from build123d import *

# Parameters (mm, degrees)
F0_W      = 56
F0_H      = 87.6
F1_DEPTH  = 5
F2_SIZE   = 2
F3_W      = 15.5
F3_H      = 25
F4_DEPTH  = 2.7
F5_R      = 3
F7_W      = 50
F7_H      = 81.6
F8_DEPTH  = 1.5
F9_R      = 1
F10_D     = 2.5
F10_DEPTH = 68
F10_START = 1.5
F10_TIP   = 0.7510757738


with BuildPart() as f1:
    # F0 (on Top) → F1 (new body)
    with BuildSketch(Plane.XY):
        Rectangle(F0_W, F0_H)
    extrude(amount=F1_DEPTH)

    # F2
    f2_edges = [f1.edges().sort_by_distance(p)[0] for p in [
        (-28, 0, 0),
    ]]
    chamfer(f2_edges, length=F2_SIZE)

    # F3 (on face) → F4 (cut)
    with BuildSketch(Plane.XY.offset(5)):
        Polygon((12.5, 43.8), (-12.5, 43.8), (-12.5, -43.8), (12.5, -43.8), (12.5, -12.5), (12.5, 12.5), align=None)
        with Locations((20.25, 0)):
            Rectangle(F3_W, F3_H)
    extrude(amount=-F4_DEPTH, mode=Mode.SUBTRACT)

    # F5
    f5_edges = [f1.edges().sort_by_distance(p)[0] for p in [
        (-28, 43.8, 3.5),
        (-28, -43.8, 3.5),
        (28, -43.8, 2.5),
        (28, 43.8, 2.5),
    ]]
    fillet(f5_edges, radius=F5_R)

    # F7 (on offset) → F8 (cut)
    with BuildSketch(Plane.XY.offset(5)):
        Rectangle(F7_W, F7_H)
    extrude(amount=-F8_DEPTH, mode=Mode.SUBTRACT)

    # F9
    f9_edges = [f1.edges().sort_by_distance(p)[0] for p in [
        (-27.12132, 42.92132, 5),
        (27.12132, 42.92132, 5),
        (18.75, 43.8, 5),
        (-18.75, 43.8, 5),
        (-28, 0, 5),
        (-18.75, -43.8, 5),
        (27.12132, -42.92132, 5),
    ]]
    fillet(f9_edges, radius=F9_R)

    # F10
    # its depths count from where the whole tool has entered the part; down to there all is cleared
    with Locations(Plane.XY.offset(5).offset(-F10_START)):
        with Locations((-20, 35.8), (20, 35.8), (20, 17.5), (20, -17.5), (20, -35.8), (-20, -35.8), (-20, 17.5), (-20, -17.5)):
            Hole(F10_D / 2, depth=F10_DEPTH)
            with Locations((0, 0, -(F10_DEPTH + F10_TIP / 2))):  # 118° drill point
                Cone(0, F10_D / 2, F10_TIP, mode=Mode.SUBTRACT)


solid = f1.part
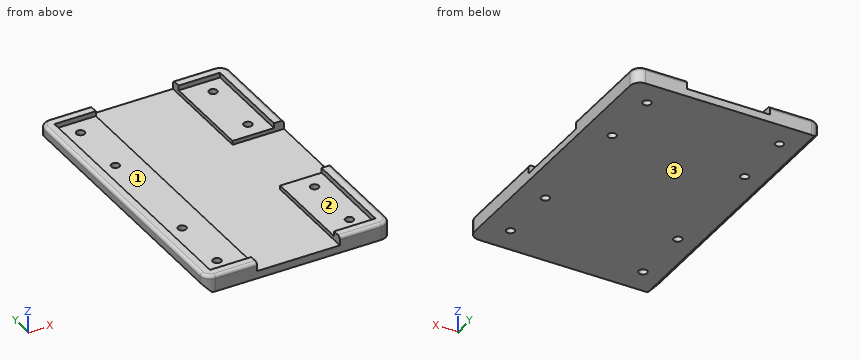
Geometry check sheet. Reference: the model listing, model coordinates, mm. Face numbers are marked on the shaded views. Round coordinates to 2 decimals unless told otherwise and drop trailing zeros. Loops run counter-clockwise (first coordinate to the right, second up) from the corner with the lowest first, then second, coordinate; pieces in that order, holes last. Notation, with made-up numbers: (69, 73.25) -> (104, 73.25) arc R16 ccw to (104, 102.25) -> close; hole circle Ø10 at (-6.5, 51.25). An arc over 180 degrees is marked (long way). Answer as a JSON object with one key per item and string values. Group by question number.
Item 1: Thickness scan on line 1 along Y through (x, z) = (20, 2.1); line 2 along X through (y, z) = (30, 2.75); line 3 along X through (y, z) = (-16.5, 3.55). Record the ranges inside material, lowest first.
Item 2: Cross-section at A-A, the plane x = -20. Record the cut outline in (y, z), plus the area to 3 significant figures.
Item 3: Cross-section at C-C, the plane y = -2. Record the cut outline in (x, z).
Item 4: Release check for a two-part mould opening along X. For the marked faces 1, 2 and 3 record: pulls with the +X half, pulls with the -X half, needs draft (parallel to the pull), parting line crosses it, or undercut.
Item 5: Cross-section at D-D, the plane x = 20. Count the separate pieces of the cut face and the enclosed holes in it, plus the area to 3 significant figures.
Item 6: Depth check by flat-ended pin: pin 1 Ø8 at (x, y) = (4.5, -2.5) entering from +Z; pin 2 Ø3 at (x, y) = (-20, -35.8) entering from +Z; pin 3 Ø2 at (y, z) = (-3.5, 4) entering from +X; pin 4 Ø1.5 at (x, y) = (20, -35.8) entering from +Z (3 decimals). Enter the tip coordinate at first touch or a pass-through.
Item 7: Cross-section at B-B, the plane y = -35.8. Record the cut outline in (x, z), plus the area to 3 significant figures.
Determined:
{
 "1": {"line 1": "y = -43.8 to -37.05, -34.55 to -18.75, -16.25 to 16.25, 18.75 to 34.55, 37.05 to 43.8", "line 2": "x = -28 to -12.5, 12.5 to 28", "line 3": "x = -28 to -25, 25 to 28"},
 "2": {"outline": "(-43.8, 0) -> (-37.05, 0) -> (-37.05, 3.5) -> (-40.8, 3.5) -> (-40.8, 5) -> (-42.8, 5) arc R1 ccw to (-43.8, 4) -> close; (-34.55, 0) -> (-18.75, 0) -> (-18.75, 3.5) -> (-34.55, 3.5) -> close; (-16.25, 0) -> (16.25, 0) -> (16.25, 3.5) -> (-16.25, 3.5) -> close; (18.75, 0) -> (34.55, 0) -> (34.55, 3.5) -> (18.75, 3.5) -> close; (37.05, 0) -> (43.8, 0) -> (43.8, 4) arc R1 ccw to (42.8, 5) -> (40.8, 5) -> (40.8, 3.5) -> (37.05, 3.5) -> close", "area": "280 mm²"},
 "3": {"outline": "(-28, 2) -> (-26, 0) -> (28, 0) -> (28, 2.3) -> (-12.5, 2.3) -> (-12.5, 3.5) -> (-25, 3.5) -> (-25, 5) -> (-27, 5) arc R1 ccw to (-28, 4) -> close"},
 "4": {"face 1": "undercut", "face 2": "undercut", "face 3": "needs draft"},
 "5": {"separate pieces": "5", "enclosed holes": "0", "area": "250 mm²"},
 "6": {"pin 1": "stops at z = 2.3", "pin 2": "stops at z = 3.5", "pin 3": "stops at x = -12.5", "pin 4": "passes through"},
 "7": {"outline": "(-28, 2) -> (-26, 0) -> (-21.25, 0) -> (-21.25, 3.5) -> (-25, 3.5) -> (-25, 5) -> (-27, 5) arc R1 ccw to (-28, 4) -> close; (-18.75, 0) -> (18.75, 0) -> (18.75, 3.5) -> (12.5, 3.5) -> (12.5, 2.3) -> (-12.5, 2.3) -> (-12.5, 3.5) -> (-18.75, 3.5) -> close; (21.25, 0) -> (28, 0) -> (28, 4) arc R1 ccw to (27, 5) -> (25, 5) -> (25, 3.5) -> (21.25, 3.5) -> close", "area": "155 mm²"}
}
